from build123d import *

# Parameters (mm, degrees)
SKETCH1_W           = 60
SKETCH1_H           = 60
BOSS_EXTRUDE1_DEPTH = 6
SKETCH2_W           = 6
SKETCH2_H           = 30
CUT_EXTRUDE1_DEPTH  = 6
SKETCH3_R           = 2
CUT_EXTRUDE2_DEPTH  = 6


with BuildPart() as part:
    # Sketch1 → Boss-Extrude1 (new body)
    with BuildSketch(Plane(origin=(0, 0, 0), x_dir=(0, 0, -1), z_dir=(1, 0, 0))):
        with Locations((30, -30)):
            Rectangle(SKETCH1_W, SKETCH1_H)
    extrude(amount=BOSS_EXTRUDE1_DEPTH)

    # Sketch2 → Cut-Extrude1 (cut)
    with BuildSketch(Plane(origin=(6, 0, 0), x_dir=(0, 0, -1), z_dir=(1, 0, 0))):
        with Locations((3, -30)):
            Rectangle(SKETCH2_W, SKETCH2_H)
        with Locations((57, -30)):
            Rectangle(SKETCH2_W, SKETCH2_H)
    extrude(amount=-CUT_EXTRUDE1_DEPTH, mode=Mode.SUBTRACT)

    # Sketch3 → Cut-Extrude2 (cut)
    with BuildSketch(Plane(origin=(6, 0, 0), x_dir=(0, 0, -1), z_dir=(1, 0, 0))):
        with Locations((18.25, -15.25)):
            Circle(SKETCH3_R)
        with Locations((41.75, -15.25)):
            Circle(SKETCH3_R)
        with Locations((41.75, -44.75)):
            Circle(SKETCH3_R)
        with Locations((18.25, -44.75)):
            Circle(SKETCH3_R)
    extrude(amount=-CUT_EXTRUDE2_DEPTH, mode=Mode.SUBTRACT)


solid = part.part
Work out the finished part from the listing and answer in its coordinate system (mm). A direction names the side the tool comes from. Give positions to 0.01 mm unless a question says otherwise; leave off trailing zeros. Order: outer loops, then holes, each group sorted by start corner. A loop starts at its lowest first (then second) coordinate and runs counter-clockwise, first axis right, second up. Notation, with made-up numbers: M 50.5,-21 L 72.5,-21 A26 cw 72.5,13 Z; hole C 30,14 d10. An arc over 180 degrees is marked long. Return JSON: item names as keys, results as strings.
Q1. The mould has two halves that part along Y. Classify faces 1 (the face through (3, 0, -30)), 2 (the face through (3, -45, -3)), 3 (the face through (3, -8, -60)): pulls with the +Y half, pulls with the -Y half, needs draft (parallel to the pull), parting line crosses it, or undercut.
Answer below:
{"face 1": "pulls with the +Y half", "face 2": "undercut", "face 3": "needs draft"}
Q2. Each of these flat-tipped pins is pushed along its axis until it touches: pin 1 (3 mm diameter, centred on y = -15.25, z = -41.75, fed in from -X); pin 2 (1.8 mm diameter, centred on x = 3, y = -24, fed in from -Z); pin 3 (1.8 mm diameter, centred on x = 3.5, y = -29.5, fed in from +Z). Where does it stop, or does it pass through?
Answer below:
{"pin 1": "passes through", "pin 2": "stops at z = -54", "pin 3": "stops at z = -6"}
Q3. Find the intervals of material crossed by line 1 along Y through (x, z) = (4.4, -41.75); line 2 along Y through (x, z) = (0.65, -3); line 3 along Z through (x, y) = (5, -29), in increasing order. Write a range as [from, to].
Answer below:
{"line 1": "y = [-60, -46.75], [-42.75, -17.25], [-13.25, 0]", "line 2": "y = [-60, -45], [-15, 0]", "line 3": "z = [-54, -6]"}
Q4. Find section B-B, the plane z = -41.75. Write down the section's boundary in (x, y).
Answer below:
{"outline": "M 0,-60 L 6,-60 L 6,-46.75 L 0,-46.75 Z; M 0,-42.75 L 6,-42.75 L 6,-17.25 L 0,-17.25 Z; M 0,-13.25 L 6,-13.25 L 6,0 L 0,0 Z"}
Q5. Which of the six approach directions +Z, -Z, +X, -X, +Y, -Y give full straight-line access (tool end or side, diameter ignored) to faces 4 (the face through (3.042, -13.267, -41.49)), 5 (the face through (3, -45, -57)), 6 (the face through (3, -30, -6))?
Answer below:
{"face 4": "+X, -X", "face 5": "-Z, +X, -X", "face 6": "+Z, +X, -X"}
Q6. Find section C-C, the plane y = -31. Write down the section's boundary in (x, z), and give its area (3 significant figures).
Answer below:
{"outline": "M 0,-54 L 6,-54 L 6,-6 L 0,-6 Z", "area": "288 mm^2"}
Q7. Find section A-A, the plane x = 4.7. Write down the section's boundary in (y, z).
Answer below:
{"outline": "M -60,-60 L -45,-60 L -45,-54 L -15,-54 L -15,-60 L 0,-60 L 0,0 L -15,0 L -15,-6 L -45,-6 L -45,0 L -60,0 Z; hole C -44.75,-41.75 d4; hole C -44.75,-18.25 d4; hole C -15.25,-41.75 d4; hole C -15.25,-18.25 d4"}
